Check sheet for the modelled part. Datum: model origin and axes. Units: mm. Coordinates: 2 decimals unless noted, no trailing zeros. Put each result on its own line as item: value.
```python
from build123d import *

# Parameters (mm, degrees)
CROQUIS1_W              = 55
CROQUIS1_H              = 70
CROQUIS1_R              = 1.5
CROQUIS1_R_2            = 2
CROQUIS1_R_3            = 3
SALIENTE_EXTRUIR1_DEPTH = 4
CHAFL_N1_SIZE           = 0.5
CHAFL_N2_SIZE           = 1.5


with BuildPart() as part:
    # Croquis1 → Saliente-Extruir1 (new body)
    with BuildSketch(Plane(origin=(0, 0, 0), x_dir=(1, 0, 0), z_dir=(0, 1, 0))):
        with Locations((19.480956658, 1.278538813)):
            Rectangle(CROQUIS1_W, CROQUIS1_H)
        with Locations(Location((6.980956658, 11.278538813, 0), (0, 0, 270))):
            Circle(CROQUIS1_R, mode=Mode.SUBTRACT)
        with Locations(Location((26.980956658, 11.278538813, 0), (0, 0, 270))):
            Circle(CROQUIS1_R, mode=Mode.SUBTRACT)
        with Locations(Location((6.980956658, -8.721461187, 0), (0, 0, 270))):
            Circle(CROQUIS1_R, mode=Mode.SUBTRACT)
        with Locations(Location((26.980956658, -8.721461187, 0), (0, 0, 270))):
            Circle(CROQUIS1_R, mode=Mode.SUBTRACT)
        with Locations(Location((31.980956658, 31.278538813, 0), (0, 0, 270))):
            Circle(CROQUIS1_R_2, mode=Mode.SUBTRACT)
        with Locations(Location((31.980956658, -28.721461187, 0), (0, 0, 270))):
            Circle(CROQUIS1_R_2, mode=Mode.SUBTRACT)
        with Locations(Location((38.480956658, -18.721461187, 0), (0, 0, 270))):
            Circle(CROQUIS1_R_2, mode=Mode.SUBTRACT)
        with Locations(Location((38.480956658, -2.521461187, 0), (0, 0, 270))):
            Circle(CROQUIS1_R_3, mode=Mode.SUBTRACT)
        with Locations(Location((38.480956658, 21.278538813, 0), (0, 0, 270))):
            Circle(CROQUIS1_R_2, mode=Mode.SUBTRACT)
    extrude(amount=SALIENTE_EXTRUIR1_DEPTH)

    # Chaflán1
    chafl_n1_edges = [part.edges().sort_by_distance(p)[0] for p in [
        (46.980956658, 4, -1.278538813),
        (6.980956658, 0, -12.778538813),
        (19.480956658, 4, -36.278538813),
        (26.980956658, 0, -12.778538813),
        (6.980956658, 0, 7.221461187),
        (26.980956658, 0, 7.221461187),
        (31.980956658, 0, -33.278538813),
        (31.980956658, 4, -33.278538813),
        (31.980956658, 0, 26.721461187),
        (31.980956658, 4, 26.721461187),
        (38.480956658, 0, 16.721461187),
        (38.480956658, 4, 16.721461187),
        (38.480956658, 0, -0.478538813),
        (38.480956658, 4, -0.478538813),
        (-8.019043342, 4, -1.278538813),
        (38.480956658, 0, -23.278538813),
        (38.480956658, 4, -23.278538813),
        (19.480956658, 0, -36.278538813),
        (46.980956658, 0, -1.278538813),
        (19.480956658, 0, 33.721461187),
        (-8.019043342, 0, -1.278538813),
        (19.480956658, 4, 33.721461187),
        (-8.019043342, 2, -36.278538813),
        (46.980956658, 2, -36.278538813),
        (46.980956658, 2, 33.721461187),
        (-8.019043342, 2, 33.721461187),
    ]]
    chamfer(chafl_n1_edges, length=CHAFL_N1_SIZE)

    # Chaflán2
    chafl_n2_edges = [part.edges().sort_by_distance(p)[0] for p in [
        (6.980956658, 4, -12.778538813),
        (26.980956658, 4, -12.778538813),
        (6.980956658, 4, 7.221461187),
        (26.980956658, 4, 7.221461187),
    ]]
    chamfer(chafl_n2_edges, length=CHAFL_N2_SIZE)


solid = part.part
```
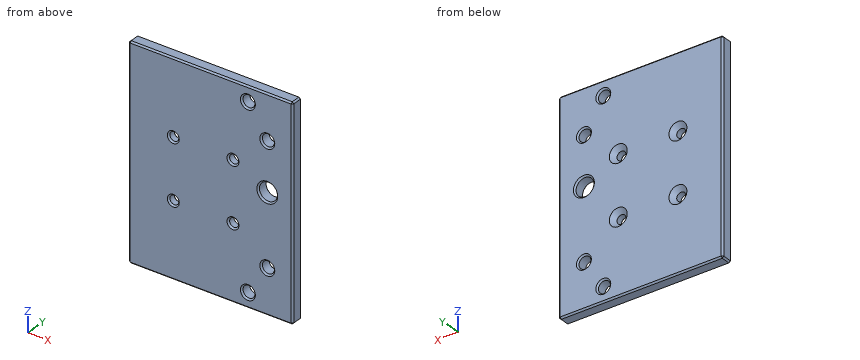
Q1. Depth check by flat-ended pin: P1, Ø2.5, axis at x = 6.98, z = -11.28, coming from the -Y side; P2, Ø3.5, axis at x = 26.98, z = 8.72, coming from the -Y side; P3, Ø4.5, axis at x = 31.98, z = 28.72, coming from the +Y side. Enter the tip coordinate at first touch or a pass-through.
Recorded:
P1: passes through
P2: stops at y = 0.25
P3: stops at y = 3.75
Q2. Material ranges on line 1 along Z through (x, y) = (40, 3.7) (3 decimals); line 2 along Z through (x, y) = (28, 2.2); line 3 along Z through (x, y) = (31, 2.25), recorded low to high.
Recorded:
line 1: z = -36.079 to -22.87, -19.687 to -0.295, 5.338 to 17.13, 20.313 to 33.521
line 2: z = -36.28 to -12.38, -10.18 to 7.62, 9.82 to 33.72
line 3: z = -36.28 to -33.02, -29.54 to 26.98, 30.46 to 33.72
Q3. Cross-section at A-A (y = 1.85). State how many separate pieces and enclosed holes the cut face has, plus the area to 3 significant figures.
Recorded:
separate pieces: 1
enclosed holes: 9
area: 3,740 mm2
